Part model, mm, in its own coordinate system. A direction names the side the tool comes from. Coordinates: 2 decimals unless noted, no trailing zeros. Loops run counter-clockwise (first coordinate to the right, second up) from the corner with the lowest first, then second, coordinate; pieces in that order, holes last. Notation, with made-up numbers: (86, 52) -> (127, 52) arc R18 cw to (127, 61) -> close; hole circle Ø3 at (-22.75, -32). An arc over 180 degrees is marked (long way). One line per item, written item: value. Start each with the question number.
from build123d import *

# Parameters (mm, degrees)
SKETCH_1_W                = 35
SKETCH_1_H                = 5
HOLE_WIZARD_1_D           = 3.4
HOLE_WIZARD_1_DEPTH       = 5
HOLE_WIZARD_2_D           = 52
HOLE_WIZARD_2_DEPTH       = 5
HOLE_WIZARD_2_CBORE_D     = 58.1
HOLE_WIZARD_2_CBORE_DEPTH = 4
SKETCH_9_R                = 1.65
CUT_EXTRUDE_1_DEPTH       = 10


with BuildPart() as part:
    # 草图1 → 旋转1 (revolve)
    with BuildSketch(Plane(origin=(0, 0, 0), x_dir=(1, 0, 0), z_dir=(0, 1, 0))):
        with Locations((17.5, 2.5)):
            Rectangle(SKETCH_1_W, SKETCH_1_H)
    revolve(axis=Axis((0, 0, -5), (0, 0, 1)))

    # 孔1
    with Locations(Plane(origin=(0, 0, -5), x_dir=(-1, 0, 0), z_dir=(0, 0, -1))):
        with Locations((16, -27.712812921), (-16, -27.712812921), (-27.712812921, -16), (-27.712812921, 16), (-16, 27.712812921), (16, 27.712812921), (27.712812921, 16), (27.712812921, -16)):
            Hole(HOLE_WIZARD_1_D / 2, depth=HOLE_WIZARD_1_DEPTH)

    # 孔2
    with Locations(Plane(origin=(0, 0, -5), x_dir=(-1, 0, 0), z_dir=(0, 0, -1))):
        with Locations((0, 0)):
            CounterBoreHole(HOLE_WIZARD_2_D / 2, HOLE_WIZARD_2_CBORE_D / 2, HOLE_WIZARD_2_CBORE_DEPTH, depth=HOLE_WIZARD_2_DEPTH)

    # 草图9 → 切除-拉伸1 (cut)
    with BuildSketch(Plane(origin=(0, 0, -5), x_dir=(-1, 0, 0), z_dir=(0, 0, -1))):
        with Locations((32, 0)):
            Circle(SKETCH_9_R)
        with Locations((0, -32)):
            Circle(SKETCH_9_R)
        with Locations((-32, 0)):
            Circle(SKETCH_9_R)
        with Locations((0, 32)):
            Circle(SKETCH_9_R)
    extrude(amount=-CUT_EXTRUDE_1_DEPTH, mode=Mode.SUBTRACT)


solid = part.part
1) Slice it at A-A (x = -16). Give the cut face in (y, z), then the cut area to 3 significant figures.
2) Tool access for faces 4 (the cylindrical face through (0.215, 33.636, -2.535)), 5 (the cylindrical face through (-26.835, -11.126, -3.028)): list every direction of +Z, -Z, +X, -X, +Y, -Y with a clear straight run to the whole face (end or side of a thin tool).
3) Slice it at B-B (y = 0). Give the cut face in (x, z), then the cut area to 3 significant figures.
4) Pin check, flat tips, straight feed: pin 1 Ø10 at (x, y) = (-8.5, 26) entering from -Z; pin 2 Ø2 at (x, z) = (4.5, -3.5) entering from -Y; pin 3 Ø1 at (y, z) = (27, -0.5) entering from +X. Stop position of each tip, or through.
5) Slice it at C-C (x = -32). Give the cut face in (y, z), then the cut area to 3 significant figures.
6) Pull direction X, two halves, no side cores. Call faces 1 (the cylindrical face through (-28, -21, -3)), 2 (the flat face through (5, 26, 0)), 3 (the flat face through (22, -15, -1)): +X half, -X half, draft (parallel to the pull), parting line (faces both ways), or undercut.
7) Probe line 1 (Y direction, x = 0, z = -2.1); line 2 (X direction, y = -27, z = -2.95); line 3 (X direction, y = -15, z = -4.4). List the from-to ranges inside material, lowest first. Write a range as from..to.
Check sheet entries:
1. outline: (-31.13, -5) -> (-29.41, -5) -> (-29.41, 0) -> (-31.13, 0) -> close; (-26.01, -5) -> (-24.25, -5) -> (-24.25, -1) -> (-20.49, -1) -> (-20.49, 0) -> (-26.01, 0) -> close; (20.49, -1) -> (24.25, -1) -> (24.25, -5) -> (26.01, -5) -> (26.01, 0) -> (20.49, 0) -> close; (29.41, -5) -> (31.13, -5) -> (31.13, 0) -> (29.41, 0) -> close
1. area: 42.3 mm^2
2. face 4: +Z, -Z
2. face 5: -Z
3. outline: (-35, -5) -> (-33.65, -5) -> (-33.65, 0) -> (-35, 0) -> close; (-30.35, -5) -> (-29.05, -5) -> (-29.05, -1) -> (-26, -1) -> (-26, 0) -> (-30.35, 0) -> close; (26, -1) -> (29.05, -1) -> (29.05, -5) -> (30.35, -5) -> (30.35, 0) -> (26, 0) -> close; (33.65, -5) -> (35, -5) -> (35, 0) -> (33.65, 0) -> close
3. area: 32.6 mm^2
4. pin 1: stops at z = -5
4. pin 2: stops at y = -34.82
4. pin 3: stops at x = 22.86
5. outline: (-14.18, -5) -> (-1.65, -5) -> (-1.65, 0) -> (-14.18, 0) -> close; (1.65, -5) -> (14.18, -5) -> (14.18, 0) -> (1.65, 0) -> close
5. area: 125 mm^2
6. face 1: parting line
6. face 2: draft
6. face 3: undercut
7. line 1: y = -35..-33.65, -30.35..-29.05, 29.05..30.35, 33.65..35
7. line 2: x = -22.27..-17.54, -14.46..-10.72, 10.72..14.46, 17.54..22.27
7. line 3: x = -31.62..-29.09, -26.34..-24.88, 24.88..26.34, 29.09..31.62
